from build123d import *

# Parameters (mm, degrees)
PAD062_DEPTH      = 7.5
PAD062_DEPTH_BACK = 7.5
POCKET036_DEPTH   = 5.5
SKETCH086_R       = 1.6
POCKET037_DEPTH   = 3.2
CHAMFER007_SIZE   = 1


with BuildPart() as part:
    # Sketch084 → Pad062 (new body, two sides)
    with BuildSketch(Plane.XZ) as pad062_sk:
        Polygon((3.5, 0), (1.75, 3.031089), (-1.75, 3.031089), (-3.5, 0), (-1.75, -3.031089), (1.75, -3.031089), align=None)
    extrude(amount=-PAD062_DEPTH)
    extrude(pad062_sk.sketch, amount=PAD062_DEPTH_BACK)

    # Sketch085 (on Face7 of Pad062) → Pocket036 (cut)
    with BuildSketch(Plane(origin=(0, 7.5, 0), x_dir=(1, 0, 0), z_dir=(0, 1, 0))):
        with BuildLine():
            Line((-1, -3.25), (1, -3.25))
            Line((1, -0.663325), (1, -3.25))
            ThreePointArc((1, -0.663325), (1.2, 0), (1, 0.663325))
            Line((1, 3.25), (1, 0.663325))
            Line((1, 3.25), (-1, 3.25))
            Line((-1, 3.25), (-1, 0.663325))
            ThreePointArc((-1, 0.663325), (-1.2, 0), (-1, -0.663325))
            Line((-1, -3.25), (-1, -0.663325))
        make_face()
    pocket036 = extrude(amount=-POCKET036_DEPTH, mode=Mode.SUBTRACT)

    # Mirrored008: Pocket036 across XZ
    add(pocket036.mirror(Plane.XZ), mode=Mode.SUBTRACT)

    # Sketch086 (on Face8 of Mirrored008) → Pocket037 (cut)
    with BuildSketch(Plane(origin=(0, 2, 0), x_dir=(1, 0, 0), z_dir=(0, 1, 0))):
        Circle(SKETCH086_R)
    pocket037 = extrude(amount=POCKET037_DEPTH, mode=Mode.SUBTRACT)

    # Mirrored009: Pocket037 across XZ
    add(pocket037.mirror(Plane.XZ), mode=Mode.SUBTRACT)

    # Chamfer007
    chamfer007_edges = [part.edges().sort_by_distance(p)[0] for p in [
        (-1.2, 7.5, 0),
        (1.2, 7.5, 0),
        (1.2, -7.5, 0),
        (-1.2, -7.5, 0),
    ]]
    chamfer(chamfer007_edges, length=CHAMFER007_SIZE)


solid = part.part
The model under review builds one solid part; all positions refer to its coordinate system, in mm. A direction names the side the tool comes from. Round coordinates to 2 decimals unless told otherwise and drop trailing zeros. Order: outer loops, then holes, each group sorted by start corner. A loop starts at its lowest first (then second) coordinate and runs counter-clockwise, first axis right, second up. Notation, with made-up numbers: (28, 85) -> (58, 85) arc R13 ccw to (58, 109) -> close; hole circle Ø2 at (-9.75, 55.5). An arc over 180 degrees is marked (long way). Use CSV: the item, a comma, the result in double quotes. Start each with the question number.
(1) Tool access review of faces 5 (the face through (-1, 5, -2)), 6 (the face through (-1.2, 5.9, 0)), 7 (the face through (-1, -5, 2)), 8 (the face through (0, -2, 0)): name each direction out of +Z, -Z, +X, -X, +Y, -Y from which nothing blocks a thin tool from reaching the whole face with its end or side.
(2) Wall thickness on probe 1 along Y at (x, z) = (0.25, -1.75); probe 2 along X at (y, z) = (4.75, 1); probe 3 along X at (y, z) = (-3.75, -1.75): over which ranges is each line inside the solid? List them lowest first. Write a range as from..to.
(3) Consider section A-A on y = 5.75. Write out the cut boundary in (x, z).
(4) Consider section B-B on y = -3. Write out the cut boundary in (x, z).
(5) Insertion check: pin 1 (2.5 mm diameter, centred on y = -3.5, z = -2.5, fed in from -X); pin 2 (1.2 mm diameter, centred on y = 5.5, z = 2, fed in from -X); pin 3 (1.6 mm diameter, centred on x = 0, z = 0, fed in from -Y); pin 4 (4 mm diameter, centred on x = 0.5, y = 6, fed in from +Z). Each pin has a flat end and moves straight along its axis. Give the tip position at first contact, or say it passes through.
(6) Consider section C-C on y = 0. Write out the cut boundary in (x, z).
(7) Consider section D-D on x = 0. Write out the cut boundary in (y, z), and give its area (3 significant figures).
(8) Mouldability with a two-part tool opening along Y and no side actions: class faces 1 (the face through (-1.6, 3.6, 0)), 2 (the face through (-1.6, -3.6, 0)), 3 (the face through (3, -7.5, 0)), 4 (the face through (-2.64, 0.11, -1.49)) as pulls with the +Y half, pulls with the -Y half, needs draft (parallel to the pull), parting line crosses it, or undercut.
Responses:
1,face 5,"+Z, -Z, +Y"
1,face 6,"+Y"
1,face 7,"+Z, -Z, -Y"
1,face 8,"none"
2,probe 1,"-2..2"
2,probe 2,"-2.92..-1.25, 1.25..2.92"
2,probe 3,"-2.49..-1, 1..2.49"
3,outline,"(-3.5, 0) -> (-1.75, -3.03) -> (-1, -3.03) -> (-1, -0.66) arc R1.2 cw to (-1, 0.66) -> (-1, 3.03) -> (-1.75, 3.03) -> close; (1, -3.03) -> (1.75, -3.03) -> (3.5, 0) -> (1.75, 3.03) -> (1, 3.03) -> (1, 0.66) arc R1.2 cw to (1, -0.66) -> close"
4,outline,"(-3.5, 0) -> (-1.75, -3.03) -> (-1, -3.03) -> (-1, -1.25) arc R1.6 cw to (-1, 1.25) -> (-1, 3.03) -> (-1.75, 3.03) -> close; (1, -3.03) -> (1.75, -3.03) -> (3.5, 0) -> (1.75, 3.03) -> (1, 3.03) -> (1, 1.25) arc R1.6 cw to (1, -1.25) -> close"
5,pin 1,"x = -2.78"
5,pin 2,"x = -2.69"
5,pin 3,"y = -2"
5,pin 4,"z = 3.03"
6,outline,"(-3.5, 0) -> (-1.75, -3.03) -> (1.75, -3.03) -> (3.5, 0) -> (1.75, 3.03) -> (-1.75, 3.03) -> close"
7,outline,"(-2, -3.03) -> (2, -3.03) -> (2, 3.03) -> (-2, 3.03) -> close"
7,area,"24.2 mm²"
8,face 1,"undercut"
8,face 2,"undercut"
8,face 3,"pulls with the -Y half"
8,face 4,"needs draft"
